```python
from build123d import *

# Parameters (mm, degrees)
F0_R     = 60
F1_DEPTH = 25
F4_DEPTH = 50.6
F5_DEPTH = 50
F6_D     = 5


with BuildPart() as f1:
    # F0 (on Front) → F1 (new body, symmetric)
    with BuildSketch(Plane.XZ):
        Circle(F0_R)
    extrude(amount=F1_DEPTH, both=True)

    # F3 (on offset) → F4 (cut, symmetric)
    with BuildSketch(Plane.XZ.offset(25)):
        with BuildLine():
            ThreePointArc((-12.654677, 2.5), (-9.062737, 8.995834), (-2.5, 12.46403))
            Line((-2.5, 12.46403), (-2.5, 56.46403))
            ThreePointArc((-2.5, 56.46403), (-40.195659, 40.137848), (-56.654677, 2.5))
            Line((-56.654677, 2.5), (-12.654677, 2.5))
        make_face()
    extrude(amount=F4_DEPTH, both=True, mode=Mode.SUBTRACT)

    # F3 (on offset) → F5 (cut, symmetric)
    with BuildSketch(Plane.XZ.offset(25)):
        with BuildLine():
            Line((-12.654677, -2.5), (-56.654677, -2.5))
            ThreePointArc((-56.654677, -2.5), (-40.195659, -40.137848), (-2.5, -56.46403))
            Line((-2.5, -56.46403), (-2.5, -12.46403))
            ThreePointArc((-2.5, -12.46403), (-9.062737, -8.995834), (-12.654677, -2.5))
        make_face()
        with BuildLine():
            ThreePointArc((12.654677, -2.5), (9.062737, -8.995834), (2.5, -12.46403))
            Line((2.5, -12.46403), (2.5, -56.46403))
            ThreePointArc((2.5, -56.46403), (40.195659, -40.137848), (56.654677, -2.5))
            Line((56.654677, -2.5), (12.654677, -2.5))
        make_face()
        with BuildLine():
            ThreePointArc((56.654677, 2.5), (40.195659, 40.137848), (2.5, 56.46403))
            Line((2.5, 56.46403), (2.5, 12.46403))
            ThreePointArc((2.5, 12.46403), (9.062737, 8.995834), (12.654677, 2.5))
            Line((12.654677, 2.5), (56.654677, 2.5))
        make_face()
    extrude(amount=F5_DEPTH, both=True, mode=Mode.SUBTRACT)

    # F6 (through all)
    with Locations(Plane.XZ.offset(25)):
        with Locations((-5, -5), (-5, 5), (5, 5), (5, -5)):
            Hole(F6_D / 2)


solid = f1.part
```
The model under review builds one solid part; all positions refer to its coordinate system, in mm. A direction names the side the tool comes from. Round coordinates to 2 decimals unless told otherwise and drop trailing zeros. Order: outer loops, then holes, each group sorted by start corner. A loop starts at its lowest first (then second) coordinate and runs counter-clockwise, first axis right, second up. Notation, with made-up numbers: M 26,8 L 75,8 A23 ccw 75,31 Z; hole C 83.5,78.5 d3. An arc over 180 degrees is marked long. Use a Markdown table: item, result.
1) Consider section A-A (z = -9). Write out the cut boundary in (x, y).
Report:
| item | result |
|---|---|
| outline | M -59.32,-25 L -56.03,-25 L -56.03,25 L -59.32,25 Z; M -9.06,-25 L 9.06,-25 L 9.06,25 L -9.06,25 Z; M 56.03,-25 L 59.32,-25 L 59.32,25 L 56.03,25 Z |
2) Tool access review of faces 5 (the face through (0, 25, 0)), 6 (the face through (-9.14, -0.35, 8.92)): name each direction out of +Z, -Z, +X, -X, +Y, -Y from which nothing blocks a thin tool from reaching the whole face with its end or side.
Report:
| item | result |
|---|---|
| face 5 | +Z, -Z, +X, -X, +Y |
| face 6 | +Y, -Y |
3) Consider section C-C (y = 0.5). Give the number of separate pieces and of enclosed holes in the cut face, then the cut area to 3 significant figures.
Report:
| item | result |
|---|---|
| separate pieces | 1 |
| enclosed holes | 8 |
| area | 2,510 mm^2 |
4) Wall thickness on line 1 along Z through (x, y) = (10.5, 17); line 2 along Z through (x, y) = (-8, 3); line 3 along Z through (x, y) = (6, -4.5): over which ranges is each line inside the solid? List them lowest first. Write a range as [from, to].
Report:
| item | result |
|---|---|
| line 1 | [-59.07, -55.62], [-7.32, 7.32], [55.62, 59.07] |
| line 2 | [-59.46, -56.01], [-9.93, 9.93], [56.01, 59.46] |
| line 3 | [-59.7, -56.24], [-11.23, -7.29], [-2.71, 2.71], [7.29, 11.23], [56.24, 59.7] |
5) Insertion check: pin 1 (22 mm diameter, centred on x = -43.5, y = -9.5, fed in from -Z); pin 2 (3 mm diameter, centred on x = -19, y = 7, fed in from +Z); pin 3 (4 mm diameter, centred on x = 5, z = -5, fed in from +Y); pin 4 (13 mm diameter, centred on x = 28.5, y = 6, fed in from -Z). Each pin has a flat end and moves straight along its axis. Give the tip position at first contact, or say it passes through.
Report:
| item | result |
|---|---|
| pin 1 | z = -50.44 |
| pin 2 | z = 57.39 |
| pin 3 | through |
| pin 4 | z = -55.82 |
6) Draft analysis for pull direction Z (two halves, no side actions). For faces 1 (the face through (-35, 0, 2.5)), 2 (the face through (-59.94, -0.35, 2.64)), 3 (the face through (2.615, 0.35, -4.249)), 4 (the face through (0, -25, 0)), state which applies: released by +Z, released by -Z, zero draft, split by the parting line, or undercut.
Report:
| item | result |
|---|---|
| face 1 | undercut |
| face 2 | split by the parting line |
| face 3 | undercut |
| face 4 | zero draft |
7) Consider section D-D (x = -5). Write out the cut boundary in (y, z), then the cut area to 3 significant figures.
Report:
| item | result |
|---|---|
| outline | M -25,-59.79 L 25,-59.79 L 25,-56.32 L -25,-56.32 Z; M -25,-11.7 L 25,-11.7 L 25,-7.5 L -25,-7.5 Z; M -25,-2.5 L 25,-2.5 L 25,2.5 L -25,2.5 Z; M -25,7.5 L 25,7.5 L 25,11.7 L -25,11.7 Z; M -25,56.32 L 25,56.32 L 25,59.79 L -25,59.79 Z |
| area | 1,020 mm^2 |
8) Consider section B-B (x = -35). Write out the cut boundary in (y, z), then the cut area to 3 significant figures.
Report:
| item | result |
|---|---|
| outline | M -25,-48.73 L 25,-48.73 L 25,-44.71 L -25,-44.71 Z; M -25,-2.5 L 25,-2.5 L 25,2.5 L -25,2.5 Z; M -25,44.71 L 25,44.71 L 25,48.73 L -25,48.73 Z |
| area | 652 mm^2 |
